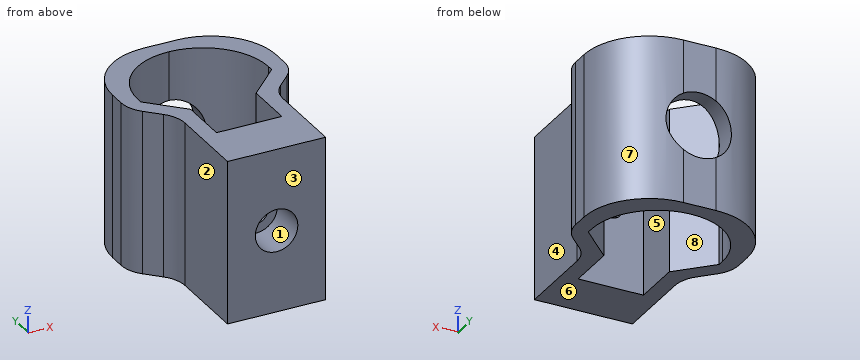
```python
from build123d import *

# Parameters (mm, degrees)
F1_DEPTH    = 25
F2_R        = 5
F3_R        = 3.25
F4_DEPTH    = 6
F5_R        = 1.85
F6_DEPTH    = 2
F7_R        = 5
F8_DEPTH    = 8.9
F9_T1_DEPTH = 75


# Not quite as in the source:
# - a fillet or chamfer that OpenCascade refuses, or shapes differently, is made with other operations: its cross-section is extruded or revolved along the edge and cut away or added


with BuildPart() as f1:
    # F0 (on Top) → F1 (new body)
    with BuildSketch(Plane.XY):
        Polygon((-7.5, 0), (0, 0), (7.5, 0), (7.5, 14.5), (12.5, 19.5), (12.5, 34), (0, 34), (-12.5, 34), (-12.5, 19.5), (-7.5, 14.5), align=None)
        with BuildLine():
            Line((-10, 20.5355339059), (-10, 21.5))
            ThreePointArc((-10, 21.5), (-7.0710678119, 28.5710678119), (0, 31.5))
            ThreePointArc((0, 31.5), (7.0710678119, 28.5710678119), (10, 21.5))
            Line((10, 21.5), (10, 20.5355339059))
            Line((10, 20.5355339059), (5, 15.5355339059))
            Line((5, 15.5355339059), (5, 8))
            Line((5, 8), (-5, 8))
            Line((-5, 8), (-5, 15.5355339059))
            Line((-5, 15.5355339059), (-10, 20.5355339059))
        make_face(mode=Mode.SUBTRACT)
    extrude(amount=F1_DEPTH)

    # F2
    f2_edges = [f1.edges().sort_by_distance(p)[0] for p in [
        (-12.5, 19.5, 12.5),
        (-7.5, 14.5, 12.5),
        (12.5, 19.5, 12.5),
        (7.5, 14.5, 12.5),
    ]]
    fillet(f2_edges, radius=F2_R)

    # F3 (on face) → F4 (cut)
    with BuildSketch(Plane.XZ):
        with Locations((0, 12.5)):
            Circle(F3_R)
    extrude(amount=-F4_DEPTH, mode=Mode.SUBTRACT)

    # F5 (on face) → F6 (cut)
    with BuildSketch(Plane(origin=(0, 8, 0), x_dir=(-1, 0, 0), z_dir=(0, 1, 0))):
        with Locations((0, 12.5)):
            Circle(F5_R)
    extrude(amount=-F6_DEPTH, mode=Mode.SUBTRACT)

    # F7 (on face) → F8 (cut)
    with BuildSketch(Plane(origin=(0, 34, 0), x_dir=(-1, 0, 0), z_dir=(0, 1, 0))):
        with Locations((0, 12.5)):
            Circle(F7_R)
    extrude(amount=-F8_DEPTH, mode=Mode.SUBTRACT)

    # F9: fillet of radius 10 on 2 edges, made by hand

    # F9_s2 → F9_t1 (cut)
    with BuildSketch(Plane.XY.offset(-25)):
        with BuildLine():
            ThreePointArc((-2.5, 34), (-9.5710678119, 31.0710678119), (-12.5, 24))
            Line((-12.5, 24), (-12.5, 34))
            Line((-12.5, 34), (-2.5, 34))
        make_face()
        with BuildLine():
            ThreePointArc((12.5, 24), (9.5710678119, 31.0710678119), (2.5, 34))
            Line((2.5, 34), (12.5, 34))
            Line((12.5, 34), (12.5, 24))
        make_face()
    extrude(amount=F9_T1_DEPTH, mode=Mode.SUBTRACT)


solid = f1.part
```
Check sheet for the modelled part. Datum: model origin and axes. Units: mm. Face numbers are marked on the shaded views. A direction names the side the tool comes from. Coordinates: 2 decimals unless noted, no trailing zeros. Write each loop counter-clockwise with the first axis right and the second up, starting at its lowest first coordinate (ties: lowest second). Pieces come first, ordered by that corner, then holes. Notation, with made-up numbers: M -29.5,13 L 20.5,13 A23 ccw 20.5,42 Z; hole C 38.25,-37 d6. An arc over 180 degrees is marked long. Use one line per item in the form item = value.
Item 1: Set-up check for the marked faces 1, 2, 3, 4 and 5: record each of +Z, -Z, +X, -X, +Y, -Y from which the full face is reachable in a straight line by a thin tool's end or side.
Answer below:
face_1 = -Y
face_2 = +Z, -Z, -X, -Y
face_3 = +Z, -Z, +X, -X, -Y
face_4 = +Z, -Z, +X, -Y
face_5 = +Z, -Z
Item 2: Material ranges on L1, parallel to Z at x = 0, y = 1.85; L2, parallel to X at y = 10.5, z = 23.25; L3, parallel to X at y = 14, z = 5, recorded low to high. Write a range as from..to.
Answer below:
L1 = 0..9.25, 15.75..25
L2 = -7.5..-5, 5..7.5
L3 = -7.75..-5, 5..7.75
Item 3: Release check for a two-part mould opening along X. For the marked faces 6, 7 and 8 record: pulls with the +X half, pulls with the -X half, needs draft (parallel to the pull), parting line crosses it, or undercut.
Answer below:
face_6 = needs draft
face_7 = pulls with the +X half
face_8 = undercut
Item 4: Sectioned sample at D-D, the plane x = 4. Record the cut outline in (y, z).
Answer below:
outline = M 0,0 L 8,0 L 8,25 L 0,25 Z; M 30.67,0 L 33.89,0 L 33.89,9.5 L 30.67,9.5 Z; M 30.67,15.5 L 33.89,15.5 L 33.89,25 L 30.67,25 Z
Item 5: Sectioned sample at A-A, the plane z = 22. Record the cut outline in (x, y).
Answer below:
outline = M -12.5,21.57 A5 ccw -11.04,18.04 L -8.96,15.96 A5 cw -7.5,12.43 L -7.5,0 L 7.5,0 L 7.5,12.43 A5 cw 8.96,15.96 L 11.04,18.04 A5 ccw 12.5,21.57 L 12.5,24 A10 ccw 2.5,34 L -2.5,34 A10 ccw -12.5,24 Z; hole M -10,20.54 L -5,15.54 L -5,8 L 5,8 L 5,15.54 L 10,20.54 L 10,21.5 A10 ccw -10,21.5 Z
Item 6: Sectioned sample at B-B, the plane x = 9.5. Record the cut outline in (y, z).
Answer below:
outline = M 16.5,0 L 20.04,0 L 20.04,25 L 16.5,25 Z; M 24.62,0 L 31.14,0 L 31.14,25 L 24.62,25 Z
Item 7: Gauge pin test, flat ends, axial feed: pin 1 Ø1 at (y, z) = (20.5, 13) entering from -X; pin 2 Ø3.5 at (y, z) = (8.5, 15) entering from -X; pin 3 Ø4.5 at (x, z) = (0, 12.5) entering from -Y. Record the tip position at first contact, or that the pin passes through.
Answer below:
pin_1 = -12.47
pin_2 = -7.5
pin_3 = 6
